Check sheet for the modelled part. Datum: model origin and axes. Units: mm. A direction names the side the tool comes from. Give positions to 0.01 mm unless a question says otherwise; leave off trailing zeros. Order: outer loops, then holes, each group sorted by start corner. A loop starts at its lowest first (then second) coordinate and runs counter-clockwise, first axis right, second up.
```python
from build123d import *

# Parameters (mm, degrees)
SKETCH1_R               = 4
BOSS_EXTRUDE1_DEPTH     = 350
SKETCH2_R               = 3
BOSS_EXTRUDE2_DEPTH     = 10
SKETCH3_R               = 1
CUT_EXTRUDE1_DEPTH      = 3
SKETCH5_R               = 4
SKETCH5_R_2             = 3
CUT_EXTRUDE3_DEPTH      = 10
SKETCH6_R               = 1
CUT_EXTRUDE4_DEPTH      = 5
CUT_EXTRUDE4_DEPTH_BACK = 5


with BuildPart() as part:
    # Sketch1 → Boss-Extrude1 (new body)
    with BuildSketch(Plane.XY):
        Circle(SKETCH1_R)
    extrude(amount=BOSS_EXTRUDE1_DEPTH)

    # Sketch2 → Boss-Extrude2 (add)
    with BuildSketch(Plane.XY.offset(350)):
        Circle(SKETCH2_R)
    extrude(amount=BOSS_EXTRUDE2_DEPTH)

    # Sketch3 → Cut-Extrude1 (cut, symmetric)
    with BuildSketch(Plane(origin=(0, 0, 0), x_dir=(1, 0, 0), z_dir=(0, 1, 0))):
        with Locations((0, -355)):
            Circle(SKETCH3_R)
    extrude(amount=CUT_EXTRUDE1_DEPTH, both=True, mode=Mode.SUBTRACT)

    # Sketch5 → Cut-Extrude3 (cut)
    with BuildSketch(Plane(origin=(0, 0, 0), x_dir=(-1, 0, 0), z_dir=(0, 0, -1))):
        Circle(SKETCH5_R)
        Circle(SKETCH5_R_2, mode=Mode.SUBTRACT)
    extrude(amount=-CUT_EXTRUDE3_DEPTH, mode=Mode.SUBTRACT)

    # Sketch6 → Cut-Extrude4 (cut, two sides)
    with BuildSketch(Plane(origin=(0, 0, 0), x_dir=(1, 0, 0), z_dir=(0, 1, 0))) as cut_extrude4_sk:
        with Locations((0, -5)):
            Circle(SKETCH6_R)
    extrude(amount=CUT_EXTRUDE4_DEPTH, mode=Mode.SUBTRACT)
    extrude(cut_extrude4_sk.sketch, amount=-CUT_EXTRUDE4_DEPTH_BACK, mode=Mode.SUBTRACT)


solid = part.part
```
Q1. Go/stop test with flat-tipped pins: P1, Ø3, axis at x = 0, z = 355, coming from the -Y side; P2, Ø2.5, axis at x = 0, z = 5, coming from the +Y side; P3, Ø1, axis at y = -2, z = 248, coming from the -X side; P4, Ø2, axis at x = -1, z = 250, coming from the -Y side. Record where each tip stops, or that it passes through.
Q2. Tool access check on faces 1 (the flat face through (0, 0, 360)), 2 (the cylindrical face through (2.77, -1.15, 354.93)), 3 (the flat face through (-1, 3, 10)). Record the directions out of +Z, -Z, +X, -X, +Y, -Y that give a thin tool (end or side, any length) a straight path to the whole face; none if there is none.
Q3. Material ranges on line 1 (Z direction, x = 0, y = -1.5); line 2 (X direction, y = -0.5, z = 355); line 3 (Z direction, x = 3, y = -2), recorded low to high.
Q4. Sectioned sample at A-A, the plane z = 267.5. Record the cut outline in (x, y), plus the area to 3 significant figures.
Q5. Sectioned sample at B-B, the plane y = -1.25. Record the cut outline in (x, z), plus the area to 3 significant figures.
Filled in:
1. P1: stops at y = -3
1. P2: stops at y = 3
1. P3: stops at x = -3.71
1. P4: stops at y = -4
2. face 1: +Z, +X, -X, +Y, -Y
2. face 2: +Z
2. face 3: -Z
3. line 1: z = 0 to 4, 6 to 354, 356 to 360
3. line 2: x = -2.96 to -1, 1 to 2.96
3. line 3: z = 10 to 350
4. outline: circle Ø8 at (0, 0)
4. area: 50.3 mm2
5. outline: (-3.8, 10) - (-2.73, 10) - (-2.73, 0) - (2.73, 0) - (2.73, 10) - (3.8, 10) - (3.8, 350) - (2.73, 350) - (2.73, 360) - (-2.73, 360) - (-2.73, 350) - (-3.8, 350) - close; hole circle Ø2 at (0, 5); hole circle Ø2 at (0, 355)
5. area: 2,690 mm2
